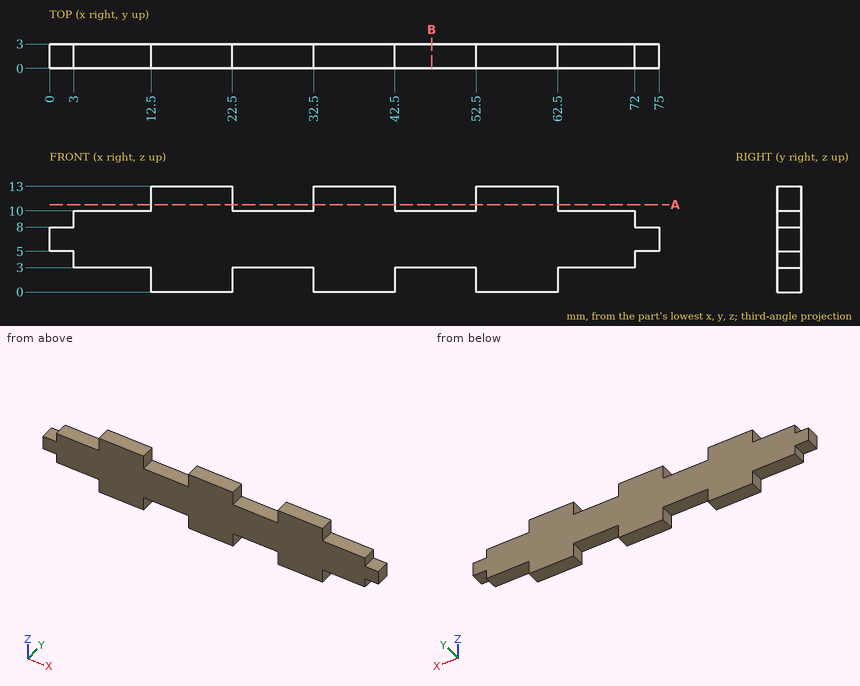
Part print with two shaded views. Sizes in mm from the minimum x, y, z corner. Round coordinates to 2 decimals unless told otherwise and drop trailing zeros. Write each loop counter-clockwise with the first axis right and the second up, starting at its lowest first coordinate (ties: lowest second). Pieces come first, ordered by that corner, then holes. Notation, with made-up numbers: (26.25, 0.25) -> (82.25, 0.25) arc R37 cw to (82.25, 36.25) -> close; hole circle Ø7 at (80.5, 66.25). An arc over 180 degrees is marked (long way). Put each result on its own line as item: value.
Item 1: Slice it at B-B, the plane x = 47. Give the cut face in (y, z), plus the area to 3 significant figures.
Here are the results:
outline: (0, 3) -> (3, 3) -> (3, 10) -> (0, 10) -> close
area: 21.0 mm^2
Item 2: Slice it at A-A, the plane z = 10.75. Give the cut face in (x, y).
Here are the results:
outline: (12.5, 0) -> (22.5, 0) -> (22.5, 3) -> (12.5, 3) -> close; (32.5, 0) -> (42.5, 0) -> (42.5, 3) -> (32.5, 3) -> close; (52.5, 0) -> (62.5, 0) -> (62.5, 3) -> (52.5, 3) -> close
Item 3: Wall check: probe 1 along X at (y, z) = (2.35, 10.5); probe 2 along X at (y, z) = (0.2, 9); probe 3 along Z at (x, y) = (66.5, 1.2). Give the ranges that are in metal, low to high. Write a range as from..to.
Here are the results:
probe 1: x = 12.5..22.5, 32.5..42.5, 52.5..62.5
probe 2: x = 3..72
probe 3: z = 3..10
Item 4: Flat gauge pins, fed straight in: P1, Ø1.5, axis at y = 2, z = 2, coming from the +X side; P2, Ø1, axis at x = 49, y = 1, coming from the -Z side; P3, Ø1.5, axis at y = 1, z = 12, coming from the -X side. Where does each tip first touch, or does it go through?
Here are the results:
P1: stops at x = 62.5
P2: stops at z = 3
P3: stops at x = 12.5
